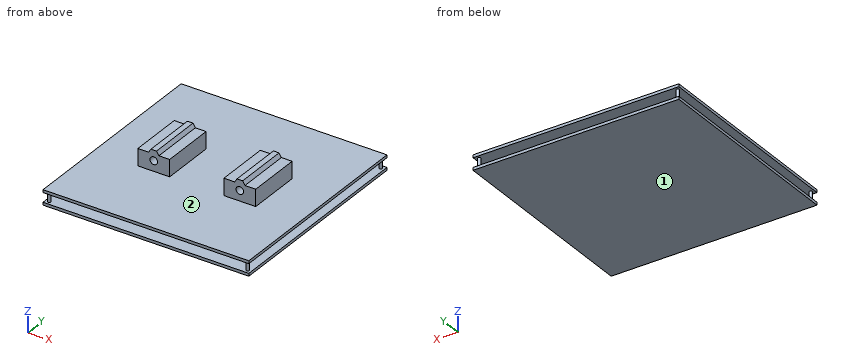
from build123d import *

# Parameters (mm, degrees)
SKETCH_1_W          = 220
SKETCH_1_H          = 220
EXTRUDE_1_DEPTH     = 3
SKETCH_2_R          = 1.5
EXTRUDE_2_DEPTH     = 10
SKETCH_3_W          = 220
SKETCH_3_H          = 220
EXTRUDE_3_DEPTH     = 3
SKETCH_4_W          = 34
SKETCH_4_H          = 58
EXTRUDE_4_DEPTH     = 22
SKETCH_5_R          = 4
CUT_EXTRUDE_1_DEPTH = 182.287065176


with BuildPart() as part:
    # 草圖1 → 填料-伸長1 (new body)
    with BuildSketch(Plane.XY):
        Rectangle(SKETCH_1_W, SKETCH_1_H)
    extrude(amount=EXTRUDE_1_DEPTH)

    # 草圖2 → 填料-伸長2 (add)
    with BuildSketch(Plane.XY.offset(3)):
        with Locations((-106, 106)):
            Circle(SKETCH_2_R)
        with Locations((106, 106)):
            Circle(SKETCH_2_R)
        with Locations((106, -106)):
            Circle(SKETCH_2_R)
        with Locations((-106, -106)):
            Circle(SKETCH_2_R)
    extrude(amount=EXTRUDE_2_DEPTH)

    # 草圖3 → 填料-伸長3 (add)
    with BuildSketch(Plane.XY.offset(13)):
        Rectangle(SKETCH_3_W, SKETCH_3_H)
    extrude(amount=EXTRUDE_3_DEPTH)

    # 草圖4 → 填料-伸長4 (add)
    with BuildSketch(Plane.XY.offset(16)):
        with Locations((-46, 0)):
            Rectangle(SKETCH_4_W, SKETCH_4_H)
    extrude_4 = extrude(amount=EXTRUDE_4_DEPTH)

    # 草圖5 → 除料-伸長1 (cut, symmetric)
    with BuildSketch(Plane(origin=(0, 29, 0), x_dir=(1, 0, 0), z_dir=(0, 1, 0))):
        with Locations(Location((-46, -27, 0), (0, 0, 270))):
            Circle(SKETCH_5_R)
        Polygon((-63, -34), (-51.5, -34), (-49, -38), (-63, -38), align=None)
        Polygon((-29, -38), (-29, -34), (-40.5, -34), (-43, -38), align=None)
    cut_extrude_1 = extrude(amount=CUT_EXTRUDE_1_DEPTH, both=True, mode=Mode.SUBTRACT)

    # 鏡射1: 填料-伸長4, 除料-伸長1 across plane
    add(extrude_4.mirror(Plane(origin=(0, 0, 0), x_dir=(0, 0, 1), z_dir=(1, 0, 0))))
    add(cut_extrude_1.mirror(Plane(origin=(0, 0, 0), x_dir=(0, 0, 1), z_dir=(1, 0, 0))), mode=Mode.SUBTRACT)


solid = part.part
Design review of the part built by this model. Coordinates are the model's own, in mm. Face numbers are marked on the shaded views. Round coordinates to 2 decimals unless told otherwise and drop trailing zeros. Loops run counter-clockwise (first coordinate to the right, second up) from the corner with the lowest first, then second, coordinate; pieces in that order, holes last. Notation, with made-up numbers: M 4.25,55 L 20.25,55 A26 cw 20.25,70 Z; hole C 68,34.5 d7. An arc over 180 degrees is marked long. Answer as a JSON object with one key per item and string values.
Item 1: We need section A-A on y = 9.5. Give the boundary of the cut face in (x, z), and give its area (3 significant figures).
Answer sheet:
{"outline": "M -110,0 L 110,0 L 110,3 L -110,3 Z; M -110,13 L 110,13 L 110,16 L 63,16 L 63,34 L 51.5,34 L 49,38 L 43,38 L 40.5,34 L 29,34 L 29,16 L -29,16 L -29,34 L -40.5,34 L -43,38 L -49,38 L -51.5,34 L -63,34 L -63,16 L -110,16 Z; hole C -46,27 d8; hole C 46,27 d8", "area": "2,510 mm^2"}
Item 2: We need section B-B on x = 76. Give the boundary of the cut face in (y, z), and give its area (3 significant figures).
Answer sheet:
{"outline": "M -110,0 L 110,0 L 110,3 L -110,3 Z; M -110,13 L 110,13 L 110,16 L -110,16 Z", "area": "1,320 mm^2"}
Item 3: We need section D-D on z = 27. Give the boundary of the cut face in (x, y), and give its area (3 significant figures).
Answer sheet:
{"outline": "M -63,-29 L -50,-29 L -50,29 L -63,29 Z; M -42,-29 L -29,-29 L -29,29 L -42,29 Z; M 29,-29 L 42,-29 L 42,29 L 29,29 Z; M 50,-29 L 63,-29 L 63,29 L 50,29 Z", "area": "3,020 mm^2"}
Item 4: Wall thickness on L1, parallel to Z at x = 46, y = -14; L2, parallel to X at y = -9, z = 27; L3, parallel to Z at x = -63, y = -87: over which ranges is each line inside the solid? List them lowest first. Write a range as from..to.
Answer sheet:
{"L1": "z = 0..3, 13..23, 31..38", "L2": "x = -63..-50, -42..-29, 29..42, 50..63", "L3": "z = 0..3, 13..16"}
Item 5: Clearance check with flat-ended pins moving along their axes: P1, Ø9, axis at x = 33.5, y = 10, coming from the +Z side; P2, Ø1.5, axis at y = 10.5, z = 28, coming from the +X side; P3, Ø9, axis at x = -46, z = 27, coming from the -Y side; P4, Ø8, axis at x = 68, z = 26, coming from the -Y side. State where each tip first meets the part, or that it passes through.
Answer sheet:
{"P1": "stops at z = 34", "P2": "stops at x = 63", "P3": "stops at y = -29", "P4": "passes through"}
Item 6: The part is to be moulded in two halves that separate along X. For the marked faces 1 and 2, say which applies: pulls with the +X half, pulls with the -X half, needs draft (parallel to the pull), parting line crosses it, or undercut.
Answer sheet:
{"face 1": "needs draft", "face 2": "undercut"}
